Check sheet for the modelled part. Datum: model origin and axes. Units: mm. A direction names the side the tool comes from. Give positions to 0.01 mm unless a question says otherwise; leave off trailing zeros. Order: outer loops, then holes, each group sorted by start corner. A loop starts at its lowest first (then second) coordinate and runs counter-clockwise, first axis right, second up.
from build123d import *

# Parameters (mm, degrees)
EXTRUDE_1_DEPTH           = 170
HOLE_WIZARD_1_D           = 11
HOLE_WIZARD_1_CBORE_D     = 18
HOLE_WIZARD_1_CBORE_DEPTH = 15
CHAMFER_1_SIZE            = 1


with BuildPart() as part:
    # 草图2 → 凸台-拉伸1 (new body)
    with BuildSketch(Plane(origin=(0, 0, 0), x_dir=(0, 0, -1), z_dir=(1, 0, 0))):
        Polygon((0, 0), (80, 0), (80, -15), (67.5, -15), (67.5, -40), (12.5, -40), (12.5, -15), (0, -15), align=None)
    extrude(amount=EXTRUDE_1_DEPTH)

    # 孔1 (through all)
    with Locations(Plane(origin=(30, 0, -40), x_dir=(0, 0, 1), z_dir=(0, 1, 0))):
        with Locations((0, 0), (0, 110)):
            CounterBoreHole(HOLE_WIZARD_1_D / 2, HOLE_WIZARD_1_CBORE_D / 2, HOLE_WIZARD_1_CBORE_DEPTH)

    # 倒角1
    chamfer_1_edges = [part.edges().sort_by_distance(p)[0] for p in [
        (85, 0, 0),
        (85, 0, -80),
    ]]
    chamfer(chamfer_1_edges, length=CHAMFER_1_SIZE)


solid = part.part
1) Material ranges on L1, parallel to X at y = -27, z = -40; L2, parallel to X at y = -10, z = -40; L3, parallel to Z at x = 29, y = -18.5, recorded low to high.
Recorded:
L1: x = 0 to 24.5, 35.5 to 134.5, 145.5 to 170
L2: x = 0 to 21, 39 to 131, 149 to 170
L3: z = -67.5 to -45.41, -34.59 to -12.5
2) Set-up check for faces 4 (the face through (34, -15, -36)), 5 (the face through (84, -15, -6)), 6 (the face through (0, -20, -41)), 7 (the face through (84, -8, 0)), 8 (the face through (84, -27, -67.5)): record each of +Z, -Z, +X, -X, +Y, -Y from which the full face is reachable in a straight line by a thin tool's end or side.
Recorded:
face 4: +Y
face 5: +Z, +X, -X, -Y
face 6: +Z, -Z, -X, +Y, -Y
face 7: +Z, +X, -X, +Y, -Y
face 8: -Z, +X, -X, -Y
3) Section check C-C, the plane y = -5.5. Record the cut outline in (x, z), then the cut area to 3 significant figures.
Recorded:
outline: (0, -80) - (170, -80) - (170, 0) - (0, 0) - close; hole circle Ø18 at (30, -40); hole circle Ø18 at (140, -40)
area: 13,100 mm2
4) Depth check by flat-ended pin: pin 1 Ø12.5 at (x, y) = (63, -28) entering from -Z; pin 2 Ø16 at (x, z) = (30, -40) entering from +Y; pin 3 Ø5 at (x, y) = (152.5, -28) entering from +Z. Enter the tip coordinate at first touch or a pass-through.
Recorded:
pin 1: stops at z = -67.5
pin 2: stops at y = -15
pin 3: stops at z = -12.5
5) Section check A-A, the plane z = -40. Record the cut outline in (x, y).
Recorded:
outline: (0, -40) - (24.5, -40) - (24.5, -15) - (21, -15) - (21, 0) - (0, 0) - close; (35.5, -40) - (134.5, -40) - (134.5, -15) - (131, -15) - (131, 0) - (39, 0) - (39, -15) - (35.5, -15) - close; (145.5, -40) - (170, -40) - (170, 0) - (149, 0) - (149, -15) - (145.5, -15) - close
6) Section check B-B, the plane x = 140. Record the cut outline in (y, z).
Recorded:
outline: (-40, -67.5) - (-15, -67.5) - (-15, -80) - (-1, -80) - (0, -79) - (0, -49) - (-15, -49) - (-15, -45.5) - (-40, -45.5) - close; (-40, -34.5) - (-15, -34.5) - (-15, -31) - (0, -31) - (0, -1) - (-1, 0) - (-15, 0) - (-15, -12.5) - (-40, -12.5) - close
7) Section check D-D, the plane x = 92.5. Record the cut outline in (y, z).
Recorded:
outline: (-40, -67.5) - (-15, -67.5) - (-15, -80) - (-1, -80) - (0, -79) - (0, -1) - (-1, 0) - (-15, 0) - (-15, -12.5) - (-40, -12.5) - close
8) Draft check along X on faces 1 (the face through (145.453, -27.675, -39.284)), 2 (the face through (170, -20, -41)), 3 (the face through (84, -28, -12.5)). Enter one of: +X half, -X half, draft (parallel to the pull), parting line (faces both ways), or undercut.
Recorded:
face 1: undercut
face 2: +X half
face 3: draft
